from build123d import *

# Parameters (mm, degrees)
SKETCH1_R             = 2.5
BOSS_EXTRUDE1_DEPTH   = 5
SKETCH1_W             = 80
SKETCH1_H             = 15
BOSS_EXTRUDE1_2_DEPTH = 5
SKETCH1_3_W           = 5
SKETCH1_3_H           = 25
BOSS_EXTRUDE2_DEPTH   = 50
CUT_EXTRUDE1_DEPTH    = 40
FILLET1_R             = 10
SKETCH3_R             = 2.5
CUT_EXTRUDE2_DEPTH    = 20
FILLET2_R             = 5


with BuildPart() as part:
    # Sketch1 → Boss-Extrude1 (new body)
    with BuildSketch(Plane(origin=(0, 0, 0), x_dir=(1, 0, 0), z_dir=(0, 1, 0))):
        with BuildLine():
            ThreePointArc((-40, -30), (-32.5, -37.5), (-25, -30))
            Line((-25, -30), (25, -30))
            ThreePointArc((25, -30), (32.5, -37.5), (40, -30))
            Line((40, -30), (40, -25))
            Line((40, -25), (35, -25))
            Line((35, -25), (35, 0))
            Line((35, 0), (35, 10))
            Line((35, 10), (-35, 10))
            Line((-35, 10), (-35, 0))
            Line((-35, 0), (-35, -25))
            Line((-35, -25), (-40, -25))
            Line((-40, -25), (-40, -30))
        make_face()
        with Locations(Location((-32.5, -30, 0), (0, 0, 270))):
            Circle(SKETCH1_R, mode=Mode.SUBTRACT)
        with Locations(Location((32.5, -30, 0), (0, 0, 270))):
            Circle(SKETCH1_R, mode=Mode.SUBTRACT)
    extrude(amount=BOSS_EXTRUDE1_DEPTH)



with BuildPart() as body_2:
    # Sketch1 → Boss-Extrude1 2 (new body)
    with BuildSketch(Plane(origin=(0, 0, 0), x_dir=(1, 0, 0), z_dir=(0, 1, 0))):
        with Locations((0, 22.5)):
            Rectangle(SKETCH1_W, SKETCH1_H)
        with Locations(Location((-32.5, 25, 0), (0, 0, 270))):
            Circle(SKETCH1_R, mode=Mode.SUBTRACT)
        with Locations(Location((32.5, 25, 0), (0, 0, 270))):
            Circle(SKETCH1_R, mode=Mode.SUBTRACT)
    extrude(amount=BOSS_EXTRUDE1_2_DEPTH)


with BuildPart() as part_1:
    add(part.part)

    add(body_2.part)  # Boss-Extrude2 merges body 2
    # Sketch1_3 → Boss-Extrude2 (add)
    with BuildSketch(Plane(origin=(0, 0, 0), x_dir=(1, 0, 0), z_dir=(0, 1, 0))):
        Polygon((-40, 15), (-40, 0), (-35, 0), (-35, 10), (35, 10), (35, 0), (40, 0), (40, 15), align=None)
        with Locations((37.5, -12.5)):
            Rectangle(SKETCH1_3_W, SKETCH1_3_H)
        with Locations((-37.5, -12.5)):
            Rectangle(SKETCH1_3_W, SKETCH1_3_H)
    extrude(amount=BOSS_EXTRUDE2_DEPTH)

    # Sketch2 → Cut-Extrude1 (cut, symmetric)
    with BuildSketch(Plane(origin=(0, 0, 0), x_dir=(0, 0, -1), z_dir=(1, 0, 0))):
        Polygon((0, 50), (-25, 5), (-25, 50), align=None)
    extrude(amount=CUT_EXTRUDE1_DEPTH, both=True, mode=Mode.SUBTRACT)

    # Fillet1
    fillet1_edges = [part_1.edges().sort_by_distance(p)[0] for p in [
        (-35, 27.5, -10),
        (35, 27.5, -10),
    ]]
    fillet(fillet1_edges, radius=FILLET1_R)

    # Sketch3 → Cut-Extrude2 (cut)
    with BuildSketch(Plane.XY):
        with Locations(Location((-22.5, 41.833761029, 0), (0, 0, 180))):
            Circle(SKETCH3_R)
        with Locations((22.5, 41.833761029)):
            Circle(SKETCH3_R)
    extrude(amount=-CUT_EXTRUDE2_DEPTH, mode=Mode.SUBTRACT)

    # Fillet2
    fillet2_edges = [part_1.edges().sort_by_distance(p)[0] for p in [
        (-25, 2.5, 30),
        (25, 2.5, 30),
    ]]
    fillet(fillet2_edges, radius=FILLET2_R)


solid = part_1.part
Here's how the part is built. I have some questions about the finished solid (model axes, mm). A direction names the side the tool comes from. Give positions to 0.01 mm unless a question says otherwise; leave off trailing zeros. Order: outer loops, then holes, each group sorted by start corner. A loop starts at its lowest first (then second) coordinate and runs counter-clockwise, first axis right, second up. Notation, with made-up numbers: (-14, 80.5) -> (38, 80.5) arc R24 cw to (38, 95.5) -> close; hole circle Ø11 at (36, 28.25). An arc over 180 degrees is marked (long way). One line per item, written item: value. Start each with the question number.
1. For faces 1 (the face through (-1, 5, -23)), 2 (the face through (32.15, 27.82, -6.99)), 3 (the face through (23.82, 2.54, 30.84)), 4 (the face through (-31, 2, -27)), which set-ups out of +Z, -Z, +X, -X, +Y, -Y let a thin tool reach every point of the face, with its end or its side?
2. We'd pull the mould along Z, two halves only. Please class faces 5 (the face through (1, 27, -15)), 6 (the face through (34, 2, 28)), 7 (the face through (-21.958, 44.274, -12.465)): released by +Z, released by -Z, zero draft, split by the parting line, or undercut.
3. Will these pins go through, and if not, where does the flat tip stop? pin 1 Ø4 at (x, y) = (-5.5, 3.5) entering from +Z; pin 2 Ø8 at (x, y) = (-22.5, 41.83) entering from +Z; pin 3 Ø2 at (x, y) = (-4.5, 32) entering from -Z.
4. Imagine slicing it at C-C, the plane x = 32.5. List the corners of the cut face in (y, z) for me.
5. Imagine slicing it at B-B, the plane x = 22.5. List the corners of the cut face in (y, z) for me.
6. Imagine slicing it at A-A, the plane z = -25. List the corners of the cut face in (x, y) for me.
7. I need wall thicknesses on probe 1 along X at (y, z) = (3.5, 31); probe 2 along X at (y, z) = (46.5, -0.5); probe 3 along Y at (x, z) = (-22.5, -11.7). Which ranges of each line are inside material? Lowest first, please. Write a range as from..to.
8. Imagine slicing it at D-D, the plane z = 24. List the corners of the cut face in (x, y) for me.
Values follow:
1. face 1: -Z, +X, -X, +Y
1. face 2: +Z, +Y
1. face 3: +Z, +Y, -Y
1. face 4: +Y, -Y
2. face 5: released by -Z
2. face 6: undercut
2. face 7: zero draft
3. pin 1: stops at z = 30
3. pin 2: stops at z = -9.89
3. pin 3: stops at z = -15
4. outline: (0, -30) -> (5, -30) -> (5, -27.5) -> (0, -27.5) -> close; (0, -22.5) -> (5, -22.5) -> (5, -15) -> (50, -15) -> (50, -6.61) -> (5, -6.61) -> (5, 27.5) -> (0, 27.5) -> close; (0, 32.5) -> (5, 32.5) -> (5, 37.5) -> (0, 37.5) -> close
5. outline: (0, -30) -> (5, -30) -> (5, -15) -> (39.33, -15) -> (39.33, -10) -> (5, -10) -> (5, 30.22) -> (0, 30.22) -> close; (44.33, -15) -> (50, -15) -> (50, -10) -> (44.33, -10) -> close
6. outline: (-40, 0) -> (-35, 0) -> (-35, 5) -> (-40, 5) -> close; (-30, 0) -> (30, 0) -> (30, 5) -> (-30, 5) -> close; (35, 0) -> (40, 0) -> (40, 5) -> (35, 5) -> close
7. probe 1: x = -39.93..-34.79, -30.21..-24.04, 24.04..30.21, 34.79..39.93
7. probe 2: x = -40..-34.99, 34.99..40
7. probe 3: y = 0..39.33, 44.33..50
8. outline: (-40, 0) -> (40, 0) -> (40, 6.8) -> (35, 6.8) -> (35, 5) -> (-35, 5) -> (-35, 6.8) -> (-40, 6.8) -> close
